Autodesk Inventor part; units mm, degrees
ref_plane "YZ Plane" through (0, 0, 0) normal (1, 0, 0) x (0, 1, 0)
ref_plane "XZ Plane" through (0, 0, 0) normal (0, 1, 0) x (-1, 0, 0)
ref_plane "XY Plane" through (0, 0, 0) normal (0, 0, 1) x (1, 0, 0)
sketch "Sketch1" plane through (0, 0, 0) normal (0, 1, 0) x (-1, 0, 0)
  line L0 (-15, 5) -> (15, 5)
  line L1 (15, 5) -> (15, -5)
  line L2 (15, -5) -> (-15, -5)
  line L3 (-15, -5) -> (-15, 5)
  dimension "d0" = 30
  dimension "d1" = 10
extrude "Extrusion1" add sketch "Sketch1" along normal blind 45
sketch "Sketch2" plane through (0, 0, 0) normal (0, -1, 0) x (1, 0, 0)
  circle A0 centre (7.5, 0) radius 1.4
  circle A1 centre (-7.5, 0) radius 1.4
  point P0 (0, 0)
  dimension "d11" = 2.8
  dimension "d12" = 2.8
extrude "Extrusion2" cut sketch "Sketch2" against normal blind 30
sketch "Sketch4" plane through (0, 45, 0) normal (0, 1, 0) x (1, 0, 0)
  circle A0 centre (0, 0) radius 1.4
  dimension "d15" = 2.8
extrude "Extrusion3" cut sketch "Sketch4" against normal blind 10
chamfer "Chamfer1" distance 5 angle 45 2 edges at (15, 45, 0) (-15, 45, 0)
chamfer "Chamfer2" distance 1 angle 45 10 edges at (15, 20, -5) (12.5, 42.5, -5) (0, 45, -5) (-12.5, 42.5, -5) (-15, 20, -5) (-15, 20, 5) (-12.5, 42.5, 5) (0, 45, 5) (12.5, 42.5, 5) (15, 20, 5)
properties part number "Side Suppor" material "ABS Plastic"
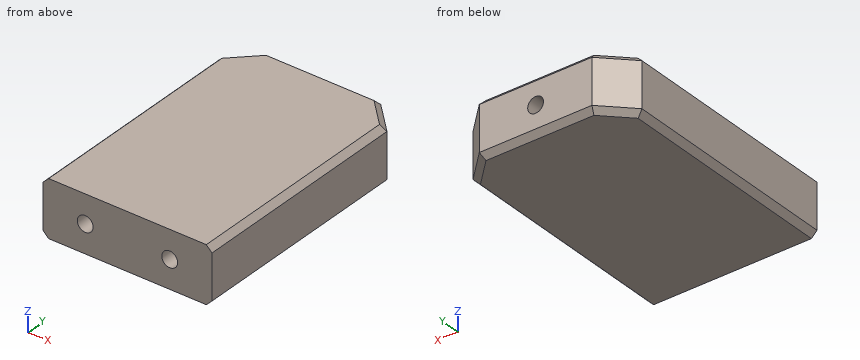
Input: part model. Units: mm. Frame: model coordinates. Coordinates: 2 decimals unless noted, no trailing zeros. Loops run counter-clockwise (first coordinate to the right, second up) from the corner with the lowest first, then second, coordinate; pieces in that order, holes last.
(1) Section A-A on y = 39. Return the cut outline in (x, z), then the cut area to 3 significant figures.
(2) First-contact query: pin 1 Ø2 at (x, z) = (7, 0.5) entering from -Y. Flat tip, straight axial feed; report the tip coordinate or a pass-through.
(3) Section D-D on y = 8. Return the cut outline in (x, z), then the cut area to 3 significant figures.
(4) Section C-C on z = 0. Return the cut outline in (x, y).
(5) Material intervals for probe 1 along Z at (x, y) = (0, 39); probe 2 along X at (y, z) = (3.5, -1.25); probe 3 along X at (y, z) = (38, 0), sorted ascending.
(6) Section B-B on x = 0. Return the cut outline in (y, z), then the cut area to 3 significant figures.
Data:
1. outline: (-15, -4) - (-14, -5) - (14, -5) - (15, -4) - (15, 4) - (14, 5) - (-14, 5) - (-15, 4) - close; hole circle Ø2.8 at (0, 0)
1. area: 292 mm2
2. pin 1: stops at y = 0
3. outline: (-15, -4) - (-14, -5) - (14, -5) - (15, -4) - (15, 4) - (14, 5) - (-14, 5) - (-15, 4) - close; hole circle Ø2.8 at (-7.5, 0); hole circle Ø2.8 at (7.5, 0)
3. area: 286 mm2
4. outline: (-15, 0) - (-8.9, 0) - (-8.9, 30) - (-6.1, 30) - (-6.1, 0) - (6.1, 0) - (6.1, 30) - (8.9, 30) - (8.9, 0) - (15, 0) - (15, 40) - (10, 45) - (1.4, 45) - (1.4, 35) - (-1.4, 35) - (-1.4, 45) - (-10, 45) - (-15, 40) - close
5. probe 1: z = -5 to -1.4, 1.4 to 5
5. probe 2: x = -15 to -8.13, -6.87 to 6.87, 8.13 to 15
5. probe 3: x = -15 to -1.4, 1.4 to 15
6. outline: (0, -5) - (44, -5) - (45, -4) - (45, -1.4) - (35, -1.4) - (35, 1.4) - (45, 1.4) - (45, 4) - (44, 5) - (0, 5) - close
6. area: 421 mm2
